from build123d import *

# Parameters (mm, degrees)
SKETCH_1_W                      = 207
SKETCH_1_H                      = 137
EXTRUDE_1_DEPTH                 = 65
SHELL_1_T                       = -1.5
SKETCH_2_R                      = 36
CUT_EXTRUDE_1_DEPTH             = 80
CUT_EXTRUDE_2_REACH             = 229.522
CUT_EXTRUDE_3_REACH             = 229.522
CUT_EXTRUDE_3_DIRECTION_2_DEPTH = 228.52197696
HOLE_WIZARD_M5_3_D              = 4.2
CUT_EXTRUDE_4_REACH             = 185.593
SKETCH_6_W                      = 160
SKETCH_6_H                      = 20


with BuildPart() as part:
    # 草图1 → 凸台-拉伸1 (new body)
    with BuildSketch(Plane.XY):
        Rectangle(SKETCH_1_W, SKETCH_1_H)
    extrude(amount=EXTRUDE_1_DEPTH)

    # 抽壳1
    shell_1_openings = [part.faces().sort_by_distance(p)[0] for p in [
        (0, 0, 65),
    ]]
    offset(amount=SHELL_1_T, openings=shell_1_openings, kind=Kind.INTERSECTION)

    # 草图2 → 切除-拉伸1 (cut)
    with BuildSketch(Plane(origin=(0, 0, 0), x_dir=(-1, 0, 0), z_dir=(0, 0, -1))):
        Circle(SKETCH_2_R)
    extrude(amount=-CUT_EXTRUDE_1_DEPTH, mode=Mode.SUBTRACT)

    # 草图4 → 切除-拉伸2 (cut, up to next)
    with BuildSketch(Plane(origin=(103.5, 0, 0), x_dir=(0, 0, -1), z_dir=(1, 0, 0)), mode=Mode.PRIVATE) as cut_extrude_2_sk1:
        with BuildLine():
            Line((-26.7, 18), (-65, 18))
            Line((-65, 18), (-65, -18))
            Line((-65, -18), (-26.7, -18))
            ThreePointArc((-26.7, -18), (-8.7, 0), (-26.7, 18))
        make_face()
    cut_extrude_2_tool1 = extrude(cut_extrude_2_sk1.sketch, amount=-CUT_EXTRUDE_2_REACH, mode=Mode.PRIVATE) & part.part
    add(cut_extrude_2_tool1.solids().sort_by_distance((103.5, 0, 38.627513))[0], mode=Mode.SUBTRACT)

    # 草图5 → 切除-拉伸3 (cut, up to next)
    with BuildSketch(Plane.ZY.offset(103.5), mode=Mode.PRIVATE) as cut_extrude_3_sk1:
        with BuildLine():
            Line((26.7, 20), (65, 20))
            Line((65, 20), (65, -20))
            Line((65, -20), (27.541433506, -19.982291902))
            ThreePointArc((27.541433506, -19.982291902), (6.704427515, -0.42080991), (26.7, 20))
        make_face()
    cut_extrude_3_tool1 = extrude(cut_extrude_3_sk1.sketch, amount=-CUT_EXTRUDE_3_REACH, mode=Mode.PRIVATE) & part.part
    add(cut_extrude_3_tool1.solids().sort_by_distance((-103.5, 0.003116, 37.811224))[0], mode=Mode.SUBTRACT)

    # 草图5 → 切除-拉伸3 direction 2 (cut)
    with BuildSketch(Plane.ZY.offset(103.5)):
        with BuildLine():
            Line((26.7, 20), (65, 20))
            Line((65, 20), (65, -20))
            Line((65, -20), (27.541433506, -19.982291902))
            ThreePointArc((27.541433506, -19.982291902), (6.704427515, -0.42080991), (26.7, 20))
        make_face()
    extrude(amount=CUT_EXTRUDE_3_DIRECTION_2_DEPTH, mode=Mode.SUBTRACT)

    # M5 螺纹槽口的螺纹槽口钻头3 (through all)
    with Locations(Plane.ZY.offset(103.5)):
        with Locations((60, 55.25), (60, -55.25)):
            Hole(HOLE_WIZARD_M5_3_D / 2)

    # 草图6 → 切除-拉伸4 (cut, up to next)
    with BuildSketch(Plane.XZ.offset(68.5), mode=Mode.PRIVATE) as cut_extrude_4_sk1:
        with Locations((0, 55)):
            Rectangle(SKETCH_6_W, SKETCH_6_H)
    cut_extrude_4_tool1 = extrude(cut_extrude_4_sk1.sketch, amount=-CUT_EXTRUDE_4_REACH, mode=Mode.PRIVATE) & part.part
    add(cut_extrude_4_tool1.solids().sort_by_distance((0, -68.5, 55))[0], mode=Mode.SUBTRACT)


solid = part.part
Input: part model. Units: mm. Frame: model coordinates. A direction names the side the tool comes from. Give positions to 0.01 mm unless a question says otherwise; leave off trailing zeros. Order: outer loops, then holes, each group sorted by start corner. A loop starts at its lowest first (then second) coordinate and runs counter-clockwise, first axis right, second up. Notation, with made-up numbers: M -1,18 L 26,18 A10 ccw 26,30 Z; hole C -13,-6 d1. An arc over 180 degrees is marked long. Answer as a JSON object with one key per item and string values.
1. Reachability of faces 5 (the cylindrical face through (102.76, 53.387, 59.031)), 6 (the flat face through (-1, 67, 33)) from +Z, -Z, +X, -X, +Y, -Y: full face, straight path, thin tool, end or side. Return the list, or none.
Result sheet:
{"face 5": "+X, -X", "face 6": "+Z"}
2. Cut plane C-C, the plane y = 0. Output: boundary loops of the cut face in (x, z), and give its area (3 significant figures).
Result sheet:
{"outline": "M -103.5,0 L -36,0 L -36,1.5 L -102,1.5 L -102,6.7 L -103.5,6.7 Z; M 36,0 L 103.5,0 L 103.5,8.7 L 102,8.7 L 102,1.5 L 36,1.5 Z", "area": "221 mm²"}
3. Pull-direction query (Y, two-part tool) for faces 1 (the flat face through (-1, 68.5, 32)), 2 (the flat face through (-102.2, -51.3, 65)), 3 (the cylindrical face through (-102.76, -0.87, 6.72)), 4 (the cylindrical face through (4.686, 35.694, 0.74)); classes: +Y half, -Y half, draft (parallel to the pull), parting line (faces both ways), or undercut.
Result sheet:
{"face 1": "+Y half", "face 2": "draft", "face 3": "undercut", "face 4": "undercut"}
4. Cut plane A-A, the plane x = 0. Output: boundary loops of the cut face in (y, z), and give its area (3 significant figures).
Result sheet:
{"outline": "M -68.5,0 L -36,0 L -36,1.5 L -67,1.5 L -67,45 L -68.5,45 Z; M 36,0 L 68.5,0 L 68.5,65 L 67,65 L 67,1.5 L 36,1.5 Z", "area": "258 mm²"}
5. First-contact query: P1, Ø3.5, axis at y = 55.25, z = 60, coming from the -X side; P2, Ø1, axis at x = -62.5, y = -10.5, coming from the +Z side; P3, Ø1.6, axis at x = -28.5, y = -68, coming from the +Z side. Flat tips, straight axial feed; report the tip coordinate or a pass-through.
Result sheet:
{"P1": "through", "P2": "z = 1.5", "P3": "z = 45"}
6. Cut plane D-D, the plane z = 23.5. Output: boundary loops of the cut face in (x, y).
Result sheet:
{"outline": "M -103.5,-68.5 L 103.5,-68.5 L 103.5,-17.71 L 102,-17.71 L 102,-67 L -102,-67 L -102,-19.74 L -103.5,-19.74 Z; M -103.5,19.74 L -102,19.74 L -102,67 L 102,67 L 102,17.71 L 103.5,17.71 L 103.5,68.5 L -103.5,68.5 Z"}
7. Cut plane B-B, the plane y = -55.25. Output: boundary loops of the cut face in (x, z), and give its area (3 significant figures).
Result sheet:
{"outline": "M -103.5,0 L 103.5,0 L 103.5,57.9 L 102,57.9 L 102,1.5 L -102,1.5 L -102,57.9 L -103.5,57.9 Z; M -103.5,62.1 L -102,62.1 L -102,65 L -103.5,65 Z; M 102,62.1 L 103.5,62.1 L 103.5,65 L 102,65 Z", "area": "488 mm²"}
8. Ray query, line 1 (Y direction, x = 103.05, z = 60); line 2 (Y direction, x = -103.1, z = 60); line 3 (Y direction, x = -41, z = 43.5). Return the intervals inside material, ascending. Write a range as [from, to].
Result sheet:
{"line 1": "[-68.5, -57.35], [-53.15, -18], [18, 53.15], [57.35, 68.5]", "line 2": "[-68.5, -57.35], [-53.15, -20], [20, 53.15], [57.35, 68.5]", "line 3": "[-68.5, -67], [67, 68.5]"}
